from build123d import *

# Parameters (mm, degrees)
SKETCH1_W                = 140
SKETCH1_H                = 30
BOSS_EXTRUDE1_DEPTH      = 80
SKETCH2_R                = 4.17592015
CUT_EXTRUDE1_DEPTH       = 15
LPATTERN1_COUNT          = 4
LPATTERN1_PITCH          = 110
SKETCH_1_R               = 25
CUT_EXTRUDE_1_DEPTH      = 10.5
SKETCH_2_R               = 5
CUT_EXTRUDE_2_DEPTH      = 10
CUT_EXTRUDE_2_DEPTH_BACK = 100
SKETCH_3_R               = 8
CUT_EXTRUDE_3_DEPTH      = 100
SKETCH_4_R               = 10
CUT_EXTRUDE_4_DEPTH      = 10.5
SKETCH_5_R               = 2.5
CUT_EXTRUDE_5_DEPTH      = 100
PATTERN_LINEAR_1_COUNT   = 2
PATTERN_LINEAR_1_PITCH   = 24
SKETCH_6_R               = 4
CUT_EXTRUDE_6_DEPTH      = 100


with BuildPart() as part:
    # Sketch1 → Boss-Extrude1 (new body)
    with BuildSketch(Plane.XY):
        with Locations((24.869684499, 8.141289438)):
            Rectangle(SKETCH1_W, SKETCH1_H)
    extrude(amount=BOSS_EXTRUDE1_DEPTH)

    # Sketch2 → Cut-Extrude1 (cut)
    with BuildSketch(Plane(origin=(0, 0, 0), x_dir=(-1, 0, 0), z_dir=(0, 0, -1))):
        with Locations((30.130315501, 7.814471991)):
            Circle(SKETCH2_R)
    cut_extrude1 = extrude(amount=-CUT_EXTRUDE1_DEPTH, mode=Mode.SUBTRACT)

    # LPattern1: Cut-Extrude1 ×4
    with Locations(*[(i * LPATTERN1_PITCH, 0, 0) for i in range(1, LPATTERN1_COUNT)]):
        add(cut_extrude1, mode=Mode.SUBTRACT)

    # Эскиз1 → Вырез-Вытянуть1 (cut)
    with BuildSketch(Plane.XZ.offset(6.858710562)):
        with Locations((-5.130315501, 33)):
            Circle(SKETCH_1_R)
    extrude(amount=-CUT_EXTRUDE_1_DEPTH, mode=Mode.SUBTRACT)

    # Эскиз2 → Вырез-Вытянуть2 (cut, two sides)
    with BuildSketch(Plane.XZ.offset(-3.641289438)) as cut_extrude_2_sk:
        with Locations((-5.130315501, 33)):
            Circle(SKETCH_2_R)
    extrude(amount=CUT_EXTRUDE_2_DEPTH, mode=Mode.SUBTRACT)
    extrude(cut_extrude_2_sk.sketch, amount=-CUT_EXTRUDE_2_DEPTH_BACK, mode=Mode.SUBTRACT)

    # Эскиз3 → Вырез-Вытянуть3 (cut)
    with BuildSketch(Plane.XZ.offset(6.858710562)):
        with Locations((-25.130315501, 52)):
            Circle(SKETCH_3_R)
    extrude(amount=-CUT_EXTRUDE_3_DEPTH, mode=Mode.SUBTRACT)

    # Эскиз4 → Вырез-Вытянуть4 (cut)
    with BuildSketch(Plane.XZ.offset(6.858710562)):
        with Locations((-25.130315501, 52)):
            Circle(SKETCH_4_R)
    extrude(amount=-CUT_EXTRUDE_4_DEPTH, mode=Mode.SUBTRACT)

    # Эскиз5 → Вырез-Вытянуть5 (cut)
    with BuildSketch(Plane(origin=(0, 23.141289438, 0), x_dir=(1, 0, 0), z_dir=(0, 1, 0))):
        with Locations((-37.130315501, -52)):
            Circle(SKETCH_5_R)
    cut_extrude_5 = extrude(amount=-CUT_EXTRUDE_5_DEPTH, mode=Mode.SUBTRACT)

    # Линейный массив1: Вырез-Вытянуть5 ×2
    with Locations(*[(i * PATTERN_LINEAR_1_PITCH, 0, 0) for i in range(1, PATTERN_LINEAR_1_COUNT)]):
        add(cut_extrude_5, mode=Mode.SUBTRACT)

    # Эскиз6 → Вырез-Вытянуть6 (cut)
    with BuildSketch(Plane(origin=(0, 23.141289438, 0), x_dir=(1, 0, 0), z_dir=(0, 1, 0))):
        with Locations((61.869684499, -48.5)):
            Circle(SKETCH_6_R)
    extrude(amount=-CUT_EXTRUDE_6_DEPTH, mode=Mode.SUBTRACT)


solid = part.part
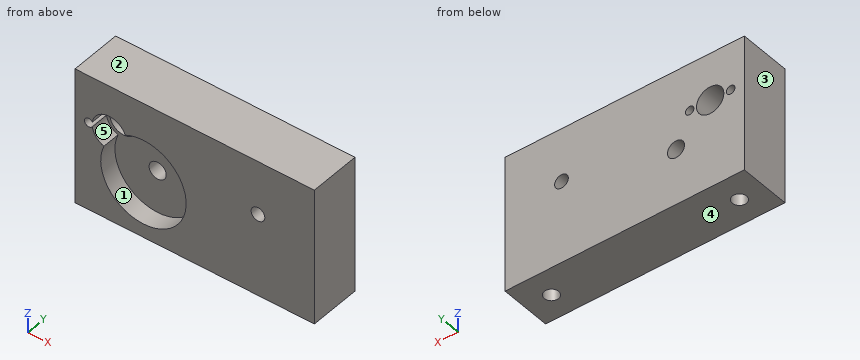
Verification items for the finished model (mm, model axes). Face numbers are marked on the shaded views. A direction names the side the tool comes from. Coordinates: 2 decimals unless noted, no trailing zeros. Loops run counter-clockwise (first coordinate to the right, second up) from the corner with the lowest first, then second, coordinate; pieces in that order, holes last. Notation, with made-up numbers: (-23, 24.5) -> (9, 24.5) arc R26 cw to (9, 52.5) -> close; hole circle Ø1 at (-29.75, 9). An arc over 180 degrees is marked (long way). Answer as a JSON object with one key per item and string values. Group by question number.
Item 1: Sectioned sample at C-C on z = 21. Record the boundary of the cut face in (x, y).
Item 2: Tool access check on the marked faces 1 and 2. Record the directions out of +Z, -Z, +X, -X, +Y, -Y that give a thin tool (end or side, any length) a straight path to the whole face; none if there is none.
Item 3: Scan lines: probe 1 along X at (y, z) = (-3.5, 33); probe 2 along X at (y, z) = (2, 52); probe 3 along X at (y, z) = (9.75, 48.5). Record each from-to range of solid material in increasing order.
Item 4: Sectioned sample at A-A on x = 61. Record the boundary of the cut face in (y, z), plus the area to 3 significant figures.
Item 5: Depth check by flat-ended pin: pin 1 (6 mm diameter, centred on x = -37.13, z = 52, fed in from -Y); pin 2 (7.5 mm diameter, centred on x = 79.87, y = 7.81, fed in from -Z). Enter the tip coordinate at first touch or a pass-through.
Item 6: Mould release check, pull along Z, two halves, no side actions. Record for the marked faces 3, 4 and 5: +Z half, -Z half, draft (parallel to the pull), parting line (faces both ways), or undercut.
Item 7: Sectioned sample at D-D on x = -13. Record the boundary of the cut face in (y, z), plus the area to 3 significant figures.
Item 8: Sectioned sample at B-B on z = 31. Record the boundary of the cut face in (x, y).
Evaluation:
{
 "1": {"outline": "(-45.13, -6.86) -> (-27.06, -6.86) -> (-27.06, 3.64) -> (16.8, 3.64) -> (16.8, -6.86) -> (94.87, -6.86) -> (94.87, 23.14) -> (-45.13, 23.14) -> close"},
 "2": {"face 1": "-Y", "face 2": "+Z, +X, -X, +Y, -Y"},
 "3": {"probe 1": "x = -45.13 to -30.13, 19.87 to 94.87", "probe 2": "x = -45.13 to -39.63, 11.12 to 59.93, 63.81 to 94.87", "probe 3": "x = -45.13 to -32.32, -17.94 to 57.87, 65.87 to 94.87"},
 "4": {"outline": "(-6.86, 0) -> (23.14, 0) -> (23.14, 44.6) -> (-6.86, 44.6) -> close; (-6.86, 52.4) -> (23.14, 52.4) -> (23.14, 80) -> (-6.86, 80) -> close", "area": "2,170 mm²"},
 "5": {"pin 1": "stops at y = -6.86", "pin 2": "stops at z = 15"},
 "6": {"face 3": "draft", "face 4": "-Z half", "face 5": "undercut"},
 "7": {"outline": "(-6.86, 0) -> (23.14, 0) -> (23.14, 49.5) -> (3.64, 49.5) -> (3.64, 9.27) -> (-6.86, 9.27) -> close; (-6.86, 56.73) -> (3.64, 56.73) -> (3.64, 54.5) -> (23.14, 54.5) -> (23.14, 80) -> (-6.86, 80) -> close", "area": "1,800 mm²"},
 "8": {"outline": "(-45.13, -6.86) -> (-30.05, -6.86) -> (-30.05, 3.64) -> (-9.71, 3.64) -> (-9.71, 23.14) -> (-45.13, 23.14) -> close; (-0.55, 3.64) -> (19.79, 3.64) -> (19.79, -6.86) -> (94.87, -6.86) -> (94.87, 23.14) -> (-0.55, 23.14) -> close"}
}
